Build history of the part. All positions in model axes, mm. A direction names the side the tool comes from. Coordinates: 2 decimals unless noted, no trailing zeros. Order: outer loops, then holes, each group sorted by start corner. A loop starts at its lowest first (then second) coordinate and runs counter-clockwise, first axis right, second up. Notation, with made-up numbers: M 64,19 L 105,19 A14 ccw 105,43 Z; hole C 73,38 d10. An arc over 180 degrees is marked long. Write item = value, one per line. Start each with the question number.
Q1. Band-saw the part on C-C on z = -38.5. Write the cut outline in (x, y).
Q2. Pull direction Z, two halves, no side cores. Call faces 1 (the face through (-66, 7, -77)), 2 (the face through (-58.114, 0.837, -27.125)), 3 (the face through (-3, 7, -3)): released by +Z, released by -Z, zero draft, split by the parting line, or undercut.
Q3. Drill centre lines: probe 1 along Z at (x, y) = (-44.2, 1.05); probe 2 along Z at (x, y) = (-10.5, 0.65); probe 3 along X at (y, z) = (-0.25, -61). Where is each one in solid material? Low to high.
Q4. Pin check, flat tips, straight feed: P1, Ø1, axis at x = -3.5, y = 7.5, coming from the -Z side; P2, Ø1.2, axis at x = -4.5, y = 8.5, coming from the +Z side; P3, Ø4, axis at x = -30, z = -56, coming from the -Y side. Stop position of each tip, or through.
Q5. Band-saw the part on A-A on y = -2.75. Write the cut outline in (x, z).
Q6. 3-axis set-ups, long thin cutter, end or side, ignore diameter. For faces 4 (the face through (-68, 7, -5)), 5 (the face through (-6, -4, -53)), 6 (the face through (-67, -4, -3)): which of +Z, -Z, +X, -X, +Y, -Y reach the whole face in a straight line?
Q7. Band-saw the part on D-D on x = -44.2. Write the cut outline in (y, z), plus the area to 3 significant figures.
Q8. Band-saw the part on B-B on x = -59.5. Write the cut outline in (y, z).
Autodesk Inventor part; units mm, degrees
ref_plane "YZ Plane" through (0, 0, 0) normal (1, 0, 0) x (0, 1, 0)
ref_plane "XZ Plane" through (0, 0, 0) normal (0, 1, 0) x (-1, 0, 0)
ref_plane "XY Plane" through (0, 0, 0) normal (0, 0, 1) x (1, 0, 0)
sketch "Sketch1" plane through (0, 0, 0) normal (0, 1, 0) x (-1, 0, 0)
  line L0 (0, 0) -> (70, 0)
  line L1 (70, 0) -> (70, -80.5)
  line L2 (70, -80.5) -> (49.49, -80.5)
  line L3 (0, 0) -> (0, -80.5)
  line L4 (0, -80.5) -> (11.33, -80.5)
  line L5 (47.54, -82.45) -> (13.28, -82.45)
  line L6 (49.49, -80.5) -> (47.54, -82.45)
  line L7 (11.33, -80.5) -> (13.28, -82.45)
  dimension "d0" = 70
  dimension "d1" = 80.5
  dimension "d2" = 20.51
  dimension "d3" = 80.5
  dimension "d4" = 11.33
  dimension "d5" = 82.45
  dimension "d6" = 45
  dimension "d7" = 45
extrude "Extrusion1" add sketch "Sketch1" along normal blind 1.65
fillet "Fillet1" radius 2 4 edges at (0, 0.825, 0) (-70, 0.825, 0) (0, 0.825, -80.5) (-70, 0.825, -80.5)
sketch "Sketch2" plane through (0, 1.65, 0) normal (0, 1, 0) x (1, 0, 0)
  circle A0 centre (-59.5, 27.7) radius 1.5
  circle A1 centre (-10.5, 29) radius 1.5
  circle A2 centre (-44.2, 80.15) radius 1.5
  line L0 (-68, 0) -> (-2, 0)
  line L1 (0, 2) -> (0, 78.5)
  line L2 (-70, 78.5) -> (-70, 2)
  line L3 (-13.28, 82.45) -> (-47.54, 82.45)
  point P0 (0, 0)
  dimension "d11" = 3
  dimension "d12" = 3
  dimension "d13" = 3
  dimension "d14" = 29
  dimension "d15" = 10.5
  dimension "d16" = 10.5
  dimension "d17" = 2.3
  dimension "d18" = 25.8
  dimension "d40" = 27.7
extrude "Extrusion2" cut sketch "Sketch2" against normal through all
sketch "Sketch3" plane through (0, 0, 0) normal (0, -1, 0) x (1, 0, 0)
  line L0 (-2, -30) -> (-6, -30)
  line L1 (-6, -30) -> (-6, -77)
  line L2 (-6, -77) -> (-2, -77)
  line L3 (-2, -77) -> (-2, -30)
  line L4 (-68, 0) -> (-2, 0)
  line L5 (0, -2) -> (0, -78.5)
  line L6 (-64, -30) -> (-68, -30)
  line L7 (-68, -30) -> (-68, -77)
  line L8 (-68, -77) -> (-64, -77)
  line L9 (-64, -77) -> (-64, -30)
  line L10 (-70, -78.5) -> (-70, -2)
  line L11 (-49.49, -80.5) -> (-68, -80.5)
  line L12 (-2, -7) -> (-4, -7)
  line L13 (-4, -7) -> (-4, -3)
  line L14 (-4, -3) -> (-2, -3)
  line L15 (-2, -3) -> (-2, -7)
  line L16 (-66, -7) -> (-68, -7)
  line L17 (-68, -7) -> (-68, -3)
  line L18 (-68, -3) -> (-66, -3)
  line L19 (-66, -3) -> (-66, -7)
  point P0 (0, 0)
  point P1 (-4, -77)
  point P2 (-66, -77)
  point P3 (-2, -5)
  point P4 (-68, -5)
  point P5 (-3, -3)
  point P6 (-67, -3)
  dimension "d21" = 4
  dimension "d22" = 47
  dimension "d23" = 30
  dimension "d24" = 2
  dimension "d27" = 2
  dimension "d28" = 4
  dimension "d30" = 30
  dimension "d33" = 2
  dimension "d34" = 4
  dimension "d35" = 2
  dimension "d36" = 4
  dimension "d37" = 3
extrude "Extrusion3" add sketch "Sketch3" along normal blind 8.3
sketch "Sketch4" plane through (0, 1.65, 0) normal (0, 1, 0) x (1, 0, 0)
  line L0 (-2, 77) -> (-2, 30)
  line L1 (-6, 30) -> (-6, 77)
  line L2 (-2, 77) -> (-6, 77)
  line L3 (-6, 77) -> (-6, 30)
  line L4 (-6, 30) -> (-2, 30)
  line L5 (-2, 30) -> (-2, 77)
  line L6 (-64, 77) -> (-64, 30)
  line L7 (-68, 77) -> (-68, 30)
  line L8 (-64, 77) -> (-68, 77)
  line L9 (-68, 77) -> (-68, 30)
  line L10 (-68, 30) -> (-64, 30)
  line L11 (-64, 30) -> (-64, 77)
  line L12 (-66, 3) -> (-66, 7)
  line L13 (-68, 3) -> (-68, 7)
  line L14 (-66, 3) -> (-68, 3)
  line L15 (-68, 3) -> (-68, 7)
  line L16 (-68, 7) -> (-66, 7)
  line L17 (-66, 7) -> (-66, 3)
  line L18 (-2, 3) -> (-2, 7)
  line L19 (-4, 7) -> (-4, 3)
  line L20 (-2, 3) -> (-4, 3)
  line L21 (-4, 3) -> (-4, 7)
  line L22 (-4, 7) -> (-2, 7)
  line L23 (-2, 7) -> (-2, 3)
  point P0 (0, 0)
extrude "Extrusion4" add sketch "Sketch4" along normal blind 10
properties part number "Microcontroller"
Recorded:
q1.outline = M -70,0 L -68,0 L -68,-8.3 L -64,-8.3 L -64,0 L -6,0 L -6,-8.3 L -2,-8.3 L -2,0 L 0,0 L 0,1.65 L -2,1.65 L -2,11.65 L -6,11.65 L -6,1.65 L -64,1.65 L -64,11.65 L -68,11.65 L -68,1.65 L -70,1.65 Z
q2.face_1 = released by -Z
q2.face_2 = undercut
q2.face_3 = released by +Z
q3.probe_1 = -82.45 to -81.65, -78.65 to 0
q3.probe_2 = -80.5 to -30.5, -27.5 to 0
q3.probe_3 = -68 to -64, -6 to -2
q4.P1 = -77
q4.P2 = -3
q4.P3 = 0
q5.outline = M -68,-77 L -64,-77 L -64,-30 L -68,-30 Z; M -68,-7 L -66,-7 L -66,-3 L -68,-3 Z; M -6,-77 L -2,-77 L -2,-30 L -6,-30 Z; M -4,-7 L -2,-7 L -2,-3 L -4,-3 Z
q6.face_4 = +Z, -Z, -X, +Y
q6.face_5 = +Z, -Z, -Y
q6.face_6 = +Z, +X, -X, -Y
q7.outline = M 0,-82.45 L 1.65,-82.45 L 1.65,-81.65 L 0,-81.65 Z; M 0,-78.65 L 1.65,-78.65 L 1.65,0 L 0,0 Z
q7.area = 131 mm2
q8.outline = M 0,-80.5 L 1.65,-80.5 L 1.65,-29.2 L 0,-29.2 Z; M 0,-26.2 L 1.65,-26.2 L 1.65,0 L 0,0 Z
